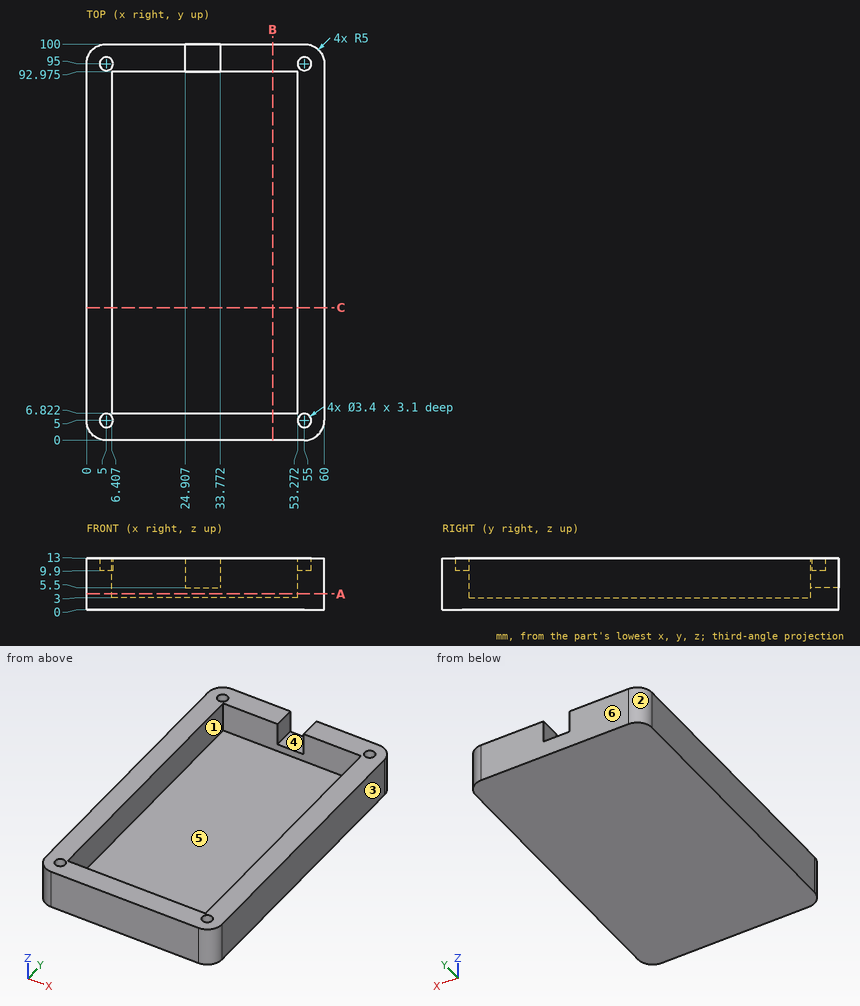
Geometry check sheet. Reference: drawing and pictorial views, mm from the part's lowest x, y, z. A direction names the side the tool comes from. Give positions to 0.01 mm unless a question says otherwise; leave off trailing zeros. Order: outer loops, then holes, each group sorted by start corner. A loop starts at its lowest first (then second) coordinate and runs counter-clockwise, first axis right, second up.
1. Access from +Z, -Z, +X, -X, +Y, -Y to the whole of each face (thin tool, end or side, straight path). Record for the marked faces 5 and 6.
2. Gauge pin test, flat ends, axial feed: pin 1 Ø2 at (y, z) = (97.5, 8) entering from +X; pin 2 Ø1 at (x, y) = (54.5, 4.5) entering from +Z; pin 3 Ø14 at (x, y) = (32, 49) entering from +Z. Record the tip position at first contact, or that the pin passes through.
3. Section check C-C, the plane y = 33.5. Enter the section's corners in (x, z).
4. Release check for a two-part mould opening along X. For the marked faces 1, 2, 3 and 4 record: pulls with the +X half, pulls with the -X half, needs draft (parallel to the pull), parting line crosses it, or undercut.
5. Thickness scan on L1, parallel to Y at x = 5, z = 12; L2, parallel to X at y = 95, z = 11.25; L3, parallel to Y at x = 46, z = 5.25 (1 decimal). Record the ranges inside material, lowest first.
6. Section check B-B, the plane x = 47. Enter the section's corners in (y, z) (1 decimal).
7. Section check A-A, the plane z = 4. Enter the section's corners in (x, y) (1 decimal), and give its area (3 significant figures).
Values follow:
1. face 5: +Z
1. face 6: +Z, -Z, +X, -X, +Y
2. pin 1: stops at x = 59.77
2. pin 2: stops at z = 9.9
2. pin 3: stops at z = 3
3. outline: (0, 0) - (60, 0) - (60, 13) - (53.27, 13) - (53.27, 3) - (6.41, 3) - (6.41, 13) - (0, 13) - close
4. face 1: undercut
4. face 2: pulls with the -X half
4. face 3: pulls with the +X half
4. face 4: undercut
5. L1: y = 0 to 3.3, 6.7 to 93.3, 96.7 to 100
5. L2: x = 0 to 3.3, 6.7 to 24.91, 33.77 to 53.3, 56.7 to 60
5. L3: y = 0 to 6.8, 93 to 100
6. outline: (0, 0) - (100, 0) - (100, 13) - (93, 13) - (93, 3) - (6.8, 3) - (6.8, 13) - (0, 13) - close
7. outline: (0, 5) arc R5 ccw to (5, 0) - (55, 0) arc R5 ccw to (60, 5) - (60, 95) arc R5 ccw to (55, 100) - (5, 100) arc R5 ccw to (0, 95) - close; hole (6.4, 6.8) - (53.3, 6.8) - (53.3, 93) - (6.4, 93) - close
7. area: 1,940 mm2
